Work out the finished part from the listing and answer in its coordinate system (mm). A direction names the side the tool comes from. Give positions to 0.01 mm unless a question says otherwise; leave off trailing zeros. Order: outer loops, then holes, each group sorted by start corner. A loop starts at its lowest first (then second) coordinate and runs counter-clockwise, first axis right, second up. Notation, with made-up numbers: (-11, 25.5) - (4, 25.5) arc R13 ccw to (4, 38.5) - close; hole circle Ø9 at (-5.75, 76). An arc over 180 degrees is marked (long way). Write each question's results on one line, items separated by ' | '.
from build123d import *

# Parameters (mm, degrees)
SKETCH2_W           = 127
SKETCH2_H           = 406.4
BOSS_EXTRUDE1_DEPTH = 3.175
SKETCH3_W           = 127
SKETCH3_H           = 3.175
BOSS_EXTRUDE2_DEPTH = 127
FILLET1_R           = 3.175
SKETCH4_R           = 2.54
CUT_EXTRUDE1_DEPTH  = 429.448574802
SKETCH5_R           = 4.7625
SKETCH5_R_2         = 2.15
CUT_EXTRUDE2_DEPTH  = 248.894110458


with BuildPart() as part:
    # Sketch2 → Boss-Extrude1 (new body)
    with BuildSketch(Plane.XY):
        Rectangle(SKETCH2_W, SKETCH2_H)
    extrude(amount=BOSS_EXTRUDE1_DEPTH)

    # Sketch3 → Boss-Extrude2 (add)
    with BuildSketch(Plane.XY.offset(3.175)):
        with Locations((0, -201.6125)):
            Rectangle(SKETCH3_W, SKETCH3_H)
    extrude(amount=BOSS_EXTRUDE2_DEPTH)

    # Fillet1
    fillet1_edges = [part.edges().sort_by_distance(p)[0] for p in [
        (0, -200.025, 3.175),
        (0, -203.2, 0),
    ]]
    fillet(fillet1_edges, radius=FILLET1_R)

    # Sketch4 → Cut-Extrude1 (cut, through all)
    with BuildSketch(Plane(origin=(0, -200.025, 0), x_dir=(1, 0, 0), z_dir=(0, 1, 0))):
        with BuildLine():
            ThreePointArc((-6.167107762, -66.675), (0.182892238, -73.025), (6.532892238, -66.675))
            Line((6.532892238, -66.675), (6.532892238, -28.575))
            ThreePointArc((6.532892238, -28.575), (0.182892238, -22.225), (-6.167107762, -28.575))
            Line((-6.167107762, -28.575), (-6.167107762, -66.675))
        make_face()
        with Locations(Location((12.7, -79.375, 0), (0, 0, 270))):
            Circle(SKETCH4_R)
        with Locations(Location((50.8, -79.375, 0), (0, 0, 270))):
            Circle(SKETCH4_R)
        with Locations(Location((50.8, -15.875, 0), (0, 0, 270))):
            Circle(SKETCH4_R)
        with Locations(Location((12.7, -15.875, 0), (0, 0, 270))):
            Circle(SKETCH4_R)
    extrude(amount=-CUT_EXTRUDE1_DEPTH, mode=Mode.SUBTRACT)

    # Sketch5 → Cut-Extrude2 (cut, through all)
    with BuildSketch(Plane.XY.offset(3.175)):
        with Locations((-50.8, 187.96)):
            Circle(SKETCH5_R)
        with Locations((50.8, 187.96)):
            Circle(SKETCH5_R)
        with Locations((-50.8, -165.1)):
            Circle(SKETCH5_R)
        with Locations((50.8, -165.1)):
            Circle(SKETCH5_R)
        with Locations((34.20875, 175.39)):
            Circle(SKETCH5_R_2)
        with Locations((4.20875, 175.39)):
            Circle(SKETCH5_R_2)
        with Locations((4.20875, 145.69)):
            Circle(SKETCH5_R_2)
        with Locations((34.20875, 145.69)):
            Circle(SKETCH5_R_2)
    extrude(amount=-CUT_EXTRUDE2_DEPTH, mode=Mode.SUBTRACT)


solid = part.part
1. A tool of negligible diameter and unlimited length cuts with its end or side. For faces 4 (the face through (-1, 6, 3.175)), 5 (the face through (-51.83, -169.75, 1.61)), from which of +Z, -Z, +X, -X, +Y, -Y can it reach the whole face along a straight path? Write none if from no direction.
Answer list:
face 4: +Z, +X, -X, +Y | face 5: +Z, -Z
2. Determine the mould class of faces 1 (the face through (-1, -200.025, 81)), 2 (the face through (-51.42, 192.68, 1.61)), 3 (the face through (-63.5, -1, 2)) for opening direction X: +X half, -X half, draft (parallel to the pull), parting line (faces both ways), or undercut.
Answer list:
face 1: draft | face 2: undercut | face 3: -X half
3. A cutting plane is placed at B-B, the plane y = -165.1. Write down the section's boundary in (x, z) (1 decimal).
Answer list:
outline: (-63.5, 0) - (-55.6, 0) - (-55.6, 3.2) - (-63.5, 3.2) - close; (-46, 0) - (46, 0) - (46, 3.2) - (-46, 3.2) - close; (55.6, 0) - (63.5, 0) - (63.5, 3.2) - (55.6, 3.2) - close
4. A cutting plane is placed at C-C, the plane x = -50.8. State how many separate pieces and enclosed holes the cut face has, then the cut area to 3 significant figures.
Answer list:
separate pieces: 3 | enclosed holes: 0 | area: 1,630 mm^2
5. Straight lines are drawn through the part: line 1 (X direction, y = 145.69, z = 0.9); line 2 (Y direction, x = -28, z = 115) (3 decimals); line 3 (Z direction, x = 50, y = -201) (3 decimals). For each, find the intervals that lie inside material, in ascending order. Write a range as [from, to].
Answer list:
line 1: [-63.5, 2.06], [6.36, 32.06], [36.36, 63.5] | line 2: [-203.2, -200.025] | line 3: [0.153, 13.464], [18.286, 76.964], [81.786, 130.175]
6. A cutting plane is placed at D-D, the plane y = -17.5. Write down the section's boundary in (x, z) (3 decimals).
Answer list:
outline: (-63.5, 0) - (63.5, 0) - (63.5, 3.175) - (-63.5, 3.175) - close
7. A cutting plane is placed at A-A, the plane z = 63. Write down the section's boundary in (x, y) (3 decimals).
Answer list:
outline: (-63.5, -203.2) - (-6.167, -203.2) - (-6.167, -200.025) - (-63.5, -200.025) - close; (6.533, -203.2) - (63.5, -203.2) - (63.5, -200.025) - (6.533, -200.025) - close
8. Given P1, Ø5.5, axis at x = 4.21, y = 145.69, coming from the -Z side; P2, Ø8, axis at x = -36.5, y = -137.5, coming from the +Z side (3 decimals); P3, Ø6.5, axis at x = 12.7, z = 79.375, coming from the +Y side (3 decimals), each flat-ended and moving along its own axis, determine where each tip first touches the part or whether it passes through.
Answer list:
P1: z = 0 | P2: z = 3.175 | P3: y = -200.025
